The model under review builds one solid part; all positions refer to its coordinate system, in mm. Coordinates: 2 decimals unless noted, no trailing zeros. Order: outer loops, then holes, each group sorted by start corner. A loop starts at its lowest first (then second) coordinate and runs counter-clockwise, first axis right, second up. Notation, with made-up numbers: (27, -17) -> (63, -17) arc R23 ccw to (63, 15) -> close; hole circle Ø6 at (75.5, 42.25). An arc over 180 degrees is marked (long way). Use one line per item in the form item = value. Start each with the question number.
(1) Take a section at B-B (y = -5.5). State the section outline as (x, z) points, then the cut area to 3 significant figures.
(2) Take a section at C-C (y = -11.5). State the section outline as (x, z) points, then the cut area to 3 significant figures.
(3) Take a section at A-A (x = -23). State the section outline as (y, z) points.
(4) Take a section at D-D (z = -7). State the section outline as (x, y) points, then the cut area to 3 significant figures.
(5) Insertion check: pin 1 Ø6 at (y, z) = (-10.5, -24) entering from -X; pin 2 Ø10 at (x, z) = (12, -19.5) entering from -Y; pin 3 Ø5 at (y, z) = (9.5, -24) entering from +X; pin 4 Ø3 at (x, y) = (13, -0.5) entering from +Z. Each pin has a flat end and moves straight along its axis. Give the tip position at first contact, or say it passes through.
(6) Mouldability with a two-part tool opening along Y and no side actions: class faces 1 (the cylindrical face through (13.069, -4.564, -15.041)), 2 (the flat face through (-17, 7, -4)), 3 (the cylindrical face through (-30.493, 0.33, -1.972)), 4 (the flat face through (-11, 15, -3)) as +Y half, -Y half, draft (parallel to the pull), parting line (faces both ways), or undercut.
(7) Wall thickness on line 1 along Y through (x, z) = (-23, -0.8); line 2 along Z through (x, y) = (-12.5, 1.75); line 3 along X through (y, z) = (-10.25, -6): over which ranges is each line inside the solid? List them lowest first.
Solid Edge part; units mm, degrees
sketch "Sketch1" plane through (0, 0, 0) normal (0, -1, 0) x (1, 0, 0)
  line L0 (0, 0) -> (-45, 0)
  line L1 (-45, 0) -> (-45, -4)
  line L2 (0, -4) -> (-45, -4)
  line L3 (26.8701, -30.8701) -> (0, -4)
  line L4 (28.8701, -28.8701) -> (26.8701, -30.8701)
  line L5 (0, 0) -> (28.8701, -28.8701)
  dimension "D1" = 45
  dimension "D2" = 26.8701
extrude "Protrusion1" add sketch "Sketch1" along normal mid plane 30
sketch "Sketch2" plane through (-15, 0, 0) normal (0, 0, 1) x (1, 0, 0)
  circle A0 centre (-8, 0) radius 7.5
  dimension "D1" = 8
extrude "Cutout1" cut sketch "Sketch2" against normal up to surface (4 mm away)
sketch "Sketch3" plane through (10.6066, 0, -10.6066) normal (0.7071068, 0, 0.7071068) x (0.7071068, 0, -0.7071068)
  circle A0 centre (10.8284, 0) radius 7.5
extrude "Cutout2" cut sketch "Sketch3" against normal up to surface (2.8284 mm away)
properties material "Stainless steel"
Findings:
q1.outline = (-45, -4) -> (-28.1, -4) -> (-28.1, 0) -> (-45, 0) -> close; (-17.9, -4) -> (0, -4) -> (12.66, -16.66) -> (14.66, -14.66) -> (0, 0) -> (-17.9, 0) -> close; (19.87, -23.87) -> (26.87, -30.87) -> (28.87, -28.87) -> (21.87, -21.87) -> close
q1.area = 222 mm²
q2.outline = (-45, -4) -> (0, -4) -> (26.87, -30.87) -> (28.87, -28.87) -> (0, 0) -> (-45, 0) -> close
q2.area = 291 mm²
q3.outline = (-15, -4) -> (-7.5, -4) -> (-7.5, 0) -> (-15, 0) -> close; (7.5, -4) -> (15, -4) -> (15, 0) -> (7.5, 0) -> close
q4.outline = (3, -15) -> (7, -15) -> (7, 15) -> (3, 15) -> close
q4.area = 120 mm²
q5.pin_1 = 17
q5.pin_2 = -15
q5.pin_3 = 26.5
q5.pin_4 = -11.5
q6.face_1 = undercut
q6.face_2 = draft
q6.face_3 = undercut
q6.face_4 = +Y half
q7.line_1 = -15 to -7.5, 7.5 to 15
q7.line_2 = -4 to 0
q7.line_3 = 2 to 6
